```python
from build123d import *


with BuildPart() as part:
    # Sketch1 → Revolve1 (revolve)
    with BuildSketch(Plane(origin=(0, 0, 0), x_dir=(0, 0, -1), z_dir=(1, 0, 0)), mode=Mode.PRIVATE) as revolve1_sk:
        with BuildLine():
            Line((-3.7, 13), (3.7, 13))
            ThreePointArc((3.7, 13), (3.912132034, 12.912132034), (4, 12.7))
            Line((4, 12.7), (4, 10.5))
            Line((4, 10.5), (2.236067977, 10.5))
            ThreePointArc((2.236067977, 10.5), (0, 11.5), (-2.236067977, 10.5))
            Line((-2.236067977, 10.5), (-4, 10.5))
            Line((-4, 10.5), (-4, 12.7))
            ThreePointArc((-4, 12.7), (-3.912132034, 12.912132034), (-3.7, 13))
        make_face()
    revolve(revolve1_sk.sketch.rotate(Axis((0, 0, 8.516129032), (0, 0, -1)), 90), axis=Axis((0, 0, 8.516129032), (0, 0, -1)))


solid = part.part
```
The model under review builds one solid part; all positions refer to its coordinate system, in mm. Give positions to 0.01 mm unless a question says otherwise; leave off trailing zeros. Write each loop counter-clockwise with the first axis right and the second up, starting at its lowest first coordinate (ties: lowest second). Pieces come first, ordered by that corner, then holes. Notation, with made-up numbers: (28.5, -0.5) - (87.5, -0.5) arc R8 ccw to (87.5, 5.5) - close; hole circle Ø5 at (7.25, -5.5). An arc over 180 degrees is marked (long way). Answer in a Markdown table with one row per item. Add a question column.
1. We need section C-C on z = 1.75. Write out the cut boundary in (x, y), then the cut area to 3 significant figures.
2. We need section D-D on z = -1.5. Write out the cut boundary in (x, y), then the cut area to 3 significant figures.
3. Wall thickness on line 1 along Y through (x, z) = (0, 3.05); line 2 along X through (y, z) = (0.75, -2.5); line 3 along X through (y, z) = (-5.5, -2): over which ranges is each line inside the solid? List them lowest first. Write a range as [from, to].
4. We need section A-A on y = 0. Write out the cut boundary in (x, z).
5. Draft analysis for pull direction X (two halves, no side actions). For faces 1 (the flat face through (8, -8, 4)), 2 (the cylindrical face through (10, -3.2, 3.1)), 3 (the cylindrical face through (10, -3.2, -3.1)), 4 (the cylindrical face through (-10.316, 7.91, -0.052)), state which applies: +X half, -X half, draft (parallel to the pull), parting line (faces both ways), or undercut.
6. Insertion check: P1, Ø1, axis at y = 7, z = -2.5, coming from the +X side; P2, Ø2, axis at y = 1, z = -2, coming from the -X side; P3, Ø12.5, axis at x = 0, y = 0, coming from the -Z side; P4, Ø1.5, axis at x = 7.5, z = 2, coming from the -Y side. Each pin has a flat end and moves straight along its axis. Give the tip position at first contact, or say it passes through.
Ans:
| question | item | result |
|---|---|---|
| 1 | outline | circle Ø26 at (0, 0); hole circle Ø21.87 at (0, 0) |
| 1 | area | 155 mm^2 |
| 2 | outline | circle Ø26 at (0, 0); hole circle Ø22.2 at (0, 0) |
| 2 | area | 144 mm^2 |
| 3 | line 1 | y = [-13, -10.5], [10.5, 13] |
| 3 | line 2 | x = [-12.98, -10.47], [10.47, 12.98] |
| 3 | line 3 | x = [-11.78, -9.22], [9.22, 11.78] |
| 4 | outline | (-13, -3.7) arc R0.3 ccw to (-12.7, -4) - (-10.5, -4) - (-10.5, -2.24) arc R3 cw to (-10.5, 2.24) - (-10.5, 4) - (-12.7, 4) arc R0.3 ccw to (-13, 3.7) - close; (10.5, -4) - (12.7, -4) arc R0.3 ccw to (13, -3.7) - (13, 3.7) arc R0.3 ccw to (12.7, 4) - (10.5, 4) - (10.5, 2.24) arc R3 cw to (10.5, -2.24) - close |
| 5 | face 1 | draft |
| 5 | face 2 | undercut |
| 5 | face 3 | undercut |
| 5 | face 4 | parting line |
| 6 | P1 | stops at x = 11.26 |
| 6 | P2 | stops at x = -13 |
| 6 | P3 | passes through |
| 6 | P4 | stops at y = -11.11 |
